```python
from build123d import *

# Parameters (mm, degrees)
F1_W     = 400
F1_H     = 400
F2_DEPTH = 25
F4_DEPTH = 400
F6_W     = 350
F6_H     = 350
F7_DEPTH = 25


with BuildPart() as f2:
    # F1 (on offset) → F2 (new body)
    with BuildSketch(Plane.XY.offset(150)):
        Rectangle(F1_W, F1_H)
    extrude(amount=-F2_DEPTH)

    # F3 (on face) → F4 (join)
    with BuildSketch(Plane(origin=(0, 0, 125), x_dir=(1, 0, 0), z_dir=(0, 0, -1))):
        Polygon((-200, 200), (-200, 150), (-175, 150), (-175, 175), (-150, 175), (-150, 200), align=None)
        Polygon((150, 175), (175, 175), (175, 150), (200, 150), (200, 200), (150, 200), align=None)
        Polygon((-150, -175), (-175, -175), (-175, -150), (-200, -150), (-200, -200), (-150, -200), align=None)
        Polygon((175, -150), (175, -175), (150, -175), (150, -200), (200, -200), (200, -150), align=None)
    extrude(amount=F4_DEPTH)

    # F6 (on offset) → F7 (join)
    with BuildSketch(Plane.XY.offset(-150)):
        Rectangle(F6_W, F6_H)
    extrude(amount=F7_DEPTH)


solid = f2.part
```
Verification items for the finished model (mm, model axes). A direction names the side the tool comes from. Give positions to 0.01 mm unless a question says otherwise; leave off trailing zeros. Loops run counter-clockwise (first coordinate to the right, second up) from the corner with the lowest first, then second, coordinate; pieces in that order, holes last. Notation, with made-up numbers: M 38,14 L 64,14 A25 ccw 64,52 Z; hole C 62.25,-27.75 d2. An arc over 180 degrees is marked long. Return JSON: item names as keys, results as strings.
1) Section check C-C, the plane z = -186.5. Enter the section's corners in (x, y).
Findings:
{"outline": "M -200,-200 L -150,-200 L -150,-175 L -175,-175 L -175,-150 L -200,-150 Z; M -200,150 L -175,150 L -175,175 L -150,175 L -150,200 L -200,200 Z; M 150,-200 L 200,-200 L 200,-150 L 175,-150 L 175,-175 L 150,-175 Z; M 150,175 L 175,175 L 175,150 L 200,150 L 200,200 L 150,200 Z"}
2) Section check A-A, the plane x = 20.5. Enter the section's corners in (y, z), and give its area (4 significant figures).
Findings:
{"outline": "M -200,125 L 200,125 L 200,150 L -200,150 Z; M -175,-150 L 175,-150 L 175,-125 L -175,-125 Z", "area": "18,750 mm2"}
3) Material ranges on L1, parallel to Z at x = -69, y = 22.5; L2, parallel to X at y = -156, z = -28.5, recorded low to high. Write a range as [from, to].
Findings:
{"L1": "z = [-150, -125], [125, 150]", "L2": "x = [-200, -175], [175, 200]"}
4) Mould release check, pull along X, two halves, no side actions. Record for faces 1 (the flat face through (175, -163, 2)), 2 (the flat face through (-200, -45, 127)), 3 (the flat face through (180, 180, -275)): released by +X, released by -X, zero draft, split by the parting line, or undercut.
Findings:
{"face 1": "undercut", "face 2": "released by -X", "face 3": "zero draft"}
5) Gauge pin test, flat ends, axial feed: P1, Ø6, axis at x = -112, y = 68.5, coming from the -Z side; P2, Ø12.5, axis at x = -62.5, z = -133, coming from the -Y side; P3, Ø7.5, axis at y = 47.5, z = -134.5, coming from the +X side. Record the tip position at first contact, or that the pin passes through.
Findings:
{"P1": "stops at z = -150", "P2": "stops at y = -175", "P3": "stops at x = 175"}
6) Section check D-D, the plane x = 159.5. Enter the section's corners in (y, z).
Findings:
{"outline": "M -200,-275 L -175,-275 L -175,-150 L 175,-150 L 175,-275 L 200,-275 L 200,150 L -200,150 Z; hole M -175,-125 L 175,-125 L 175,125 L -175,125 Z"}
7) Tool access check on faces 4 (the flat face through (-163, -175, -212)), 5 (the flat face through (-175, -2, -138)), 6 (the flat face through (-163, -175, 2)), 7 (the flat face through (-2, 175, -138)). Record the directions out of +Z, -Z, +X, -X, +Y, -Y that give a thin tool (end or side, any length) a straight path to the whole face; none if there is none.
Findings:
{"face 4": "-Z", "face 5": "-Z, -X", "face 6": "none", "face 7": "-Z, +Y"}
